Design review of the part shown in the three views and the two pictorial views. Dimensions are in mm from the part's minimum x, y and z. A direction names the side the tool comes from. Round coordinates to 2 decimals unless told otherwise and drop trailing zeros. Write each loop counter-clockwise with the first axis right and the second up, starting at its lowest first coordinate (ties: lowest second). Pieces come first, ordered by that corner, then holes. Notation, with made-up numbers: (24.5, -22) -> (75.5, -22) arc R21 ccw to (75.5, 16) -> close; hole circle Ø4 at (-13, 10). An arc over 180 degrees is marked (long way). One line per question, with ' | ' between items. Start each with the question number.
1) Consider section C-C (z = 10). Give the boundary of the cut face in (x, y).
2) For probe 1 along Y at (x, z) = (33, 13.25); probe 2 along X at (y, z) = (26.5, 13); probe 3 along Y at (x, z) = (54.5, 3.75), list the stretches that pass through material, from the lowest coordinate up.
3) For the marked faces 1 and 2, list the 3-axis set-ups (+Z, -Z, +X, -X, +Y, -Y) from which the entire face can be reached by the end or side of a thin tool; tool diameter is ignored.
4) Consider section A-A (x = 84). Give the boundary of the cut face in (y, z), then the cut area to 3 significant figures.
5) Insertion check: pin 1 Ø4 at (x, z) = (91, 14.5) entering from -Y; pin 2 Ø8 at (x, y) = (61.5, 31) entering from -Z; pin 3 Ø4 at (x, z) = (63, 7) entering from -Y. Each pin has a flat end and moves straight along its axis. Give the tip position at first contact, or say it passes through.
6) Consider section B-B (y = 28). Give the boundary of the cut face in (x, z).
7) Consider section D-D (x = 54). Give the boundary of the cut face in (y, z).
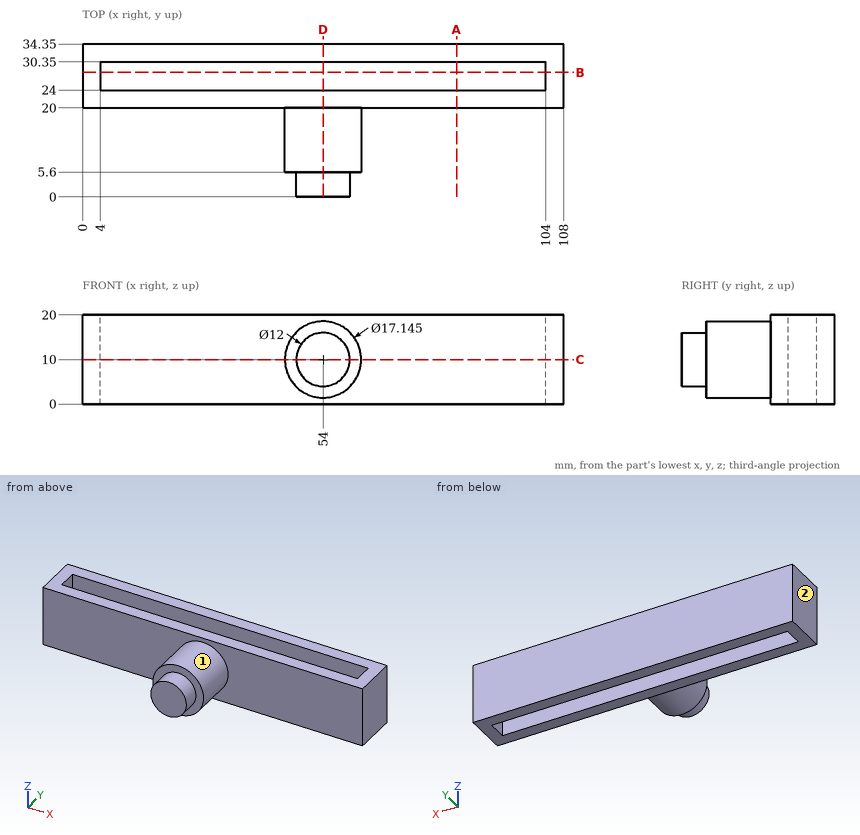
From the geometry:
1) outline: (0, 20) -> (45.43, 20) -> (45.43, 5.6) -> (48, 5.6) -> (48, 0) -> (60, 0) -> (60, 5.6) -> (62.57, 5.6) -> (62.57, 20) -> (108, 20) -> (108, 34.35) -> (0, 34.35) -> close; hole (4, 24) -> (104, 24) -> (104, 30.35) -> (4, 30.35) -> close
2) probe 1: y = 20 to 24, 30.35 to 34.35 | probe 2: x = 0 to 4, 104 to 108 | probe 3: y = 5.6 to 24, 30.35 to 34.35
3) face 1: -Y | face 2: +Z, -Z, -X, +Y, -Y
4) outline: (20, 0) -> (24, 0) -> (24, 20) -> (20, 20) -> close; (30.35, 0) -> (34.35, 0) -> (34.35, 20) -> (30.35, 20) -> close | area: 160 mm2
5) pin 1: stops at y = 20 | pin 2: stops at z = 0 | pin 3: stops at y = 5.6
6) outline: (0, 0) -> (4, 0) -> (4, 20) -> (0, 20) -> close; (104, 0) -> (108, 0) -> (108, 20) -> (104, 20) -> close
7) outline: (0, 4) -> (5.6, 4) -> (5.6, 1.43) -> (20, 1.43) -> (20, 0) -> (24, 0) -> (24, 20) -> (20, 20) -> (20, 18.57) -> (5.6, 18.57) -> (5.6, 16) -> (0, 16) -> close; (30.35, 0) -> (34.35, 0) -> (34.35, 20) -> (30.35, 20) -> close
